```python
from build123d import *

# Parameters (mm, degrees)
SKETCH2_W           = 1006.2
SKETCH2_H           = 425
SKETCH2_W_2         = 1003.025
SKETCH2_H_2         = 421.825
BOSS_EXTRUDE1_DEPTH = 420
BOSS_EXTRUDE2_START = 420
SKETCH3_W           = 1006.2
SKETCH3_H           = 425
BOSS_EXTRUDE2_DEPTH = 1.5875
FILLET2_R           = 5
CUT_EXTRUDE1_REACH  = 1112.853
SKETCH4_W           = 80
SKETCH4_H           = 80
SKETCH7_W           = 57.15
SKETCH7_H           = 57.15
CUT_EXTRUDE2_DEPTH  = 420
SKETCH8_W           = 180
SKETCH8_H           = 100
CUT_EXTRUDE3_DEPTH  = 503.1
SKETCH9_W           = 180
SKETCH9_H           = 100
CUT_EXTRUDE4_DEPTH  = 503.1


with BuildPart() as part:
    # Sketch2 → Boss-Extrude1 (new body)
    with BuildSketch(Plane(origin=(0, 0, 0), x_dir=(1, 0, 0), z_dir=(0, 1, 0))):
        Rectangle(SKETCH2_W, SKETCH2_H)
        Rectangle(SKETCH2_W_2, SKETCH2_H_2, mode=Mode.SUBTRACT)
    extrude(amount=BOSS_EXTRUDE1_DEPTH)

    # Sketch3 → Boss-Extrude2 (add)
    with BuildSketch(Plane(origin=(0, 0, 0), x_dir=(1, 0, 0), z_dir=(0, 1, 0)).offset(BOSS_EXTRUDE2_START)):
        Rectangle(SKETCH3_W, SKETCH3_H)
    extrude(amount=-BOSS_EXTRUDE2_DEPTH)

    # Fillet2
    fillet2_edges = [part.edges().sort_by_distance(p)[0] for p in [
        (-503.1, 420, 0),
        (0, 420, 212.5),
        (503.1, 420, 0),
        (503.1, 210, 212.5),
        (-503.1, 210, 212.5),
        (-503.1, 210, -212.5),
        (503.1, 210, -212.5),
        (0, 420, -212.5),
    ]]
    fillet(fillet2_edges, radius=FILLET2_R)

    # Sketch4 → Cut-Extrude1 (cut, up to next)
    with BuildSketch(Plane.ZY.offset(503.1), mode=Mode.PRIVATE) as cut_extrude1_sk1:
        with Locations((0, 40)):
            Rectangle(SKETCH4_W, SKETCH4_H)
    cut_extrude1_tool1 = extrude(cut_extrude1_sk1.sketch, amount=-CUT_EXTRUDE1_REACH, mode=Mode.PRIVATE) & part.part
    add(cut_extrude1_tool1.solids().sort_by_distance((-503.1, 40, 0))[0], mode=Mode.SUBTRACT)

    # Sketch7 → Cut-Extrude2 (cut)
    with BuildSketch(Plane(origin=(0, 0, 0), x_dir=(1, 0, 0), z_dir=(0, 1, 0))):
        with Locations((220.4, 0)):
            Rectangle(SKETCH7_W, SKETCH7_H)
    extrude(amount=CUT_EXTRUDE2_DEPTH, mode=Mode.SUBTRACT)

    # Sketch8 → Cut-Extrude3 (cut)
    with BuildSketch(Plane(origin=(0, 0, 0), x_dir=(0, 0, -1), z_dir=(1, 0, 0))):
        with Locations((0, 330)):
            Rectangle(SKETCH8_W, SKETCH8_H)
    extrude(amount=CUT_EXTRUDE3_DEPTH, mode=Mode.SUBTRACT)

    # Sketch9 → Cut-Extrude4 (cut)
    with BuildSketch(Plane(origin=(0, 0, 0), x_dir=(0, 0, -1), z_dir=(1, 0, 0))):
        with Locations((0, 130)):
            Rectangle(SKETCH9_W, SKETCH9_H)
    extrude(amount=-CUT_EXTRUDE4_DEPTH, mode=Mode.SUBTRACT)


solid = part.part
```
Verification items for the finished model (mm, model axes). A direction names the side the tool comes from. Give positions to 0.01 mm unless a question says otherwise; leave off trailing zeros. Loops run counter-clockwise (first coordinate to the right, second up) from the corner with the lowest first, then second, coordinate; pieces in that order, holes last.
1. Section check A-A, the plane z = -74. Enter the section's corners in (x, y).
2. Section check B-B, the plane y = 139.5. Enter the section's corners in (x, z).
3. Section check D-D, the plane z = 155.5. Enter the section's corners in (x, y).
4. Thickness scan on line 1 (Z direction, x = 170.5, y = 35); line 2 (X direction, y = 65.5, z = 175); line 3 (Y direction, x = -453.5, z = -153). Record the ranges inside material, lowest first.
5. Set-up check for faces 4 (the flat face through (-7, 205, -212.5)), 5 (the flat face through (501.512, 206, 3)): record each of +Z, -Z, +X, -X, +Y, -Y from which the full face is reachable in a straight line by a thin tool's end or side.
6. Mould release check, pull along X, two halves, no side actions. Record for faces 1 (the flat face through (-7, 206, 210.912)), 2 (the flat face through (503.1, 205, 3)), 3 (the flat face through (-7, 205, 212.5)): released by +X, released by -X, zero draft, split by the parting line, or undercut.
7. Section check C-C, the plane x = -287.5. Enter the section's corners in (y, z), then the cut area to 3 significant figures.
8. Go/stop test with flat-tipped pins: pin 1 Ø0.8 at (x, z) = (502.5, -39) entering from +Y; pin 2 Ø0.8 at (x, z) = (-502, 63) entering from +Y; pin 3 Ø3 at (x, z) = (-350.5, 15) entering from -Y. Record where each tip stops, or that it passes through.
Geometry says:
1. outline: (-503.1, 0) - (-501.51, 0) - (-501.51, 80) - (-503.1, 80) - close; (-503.1, 180) - (-501.51, 180) - (-501.51, 418.41) - (501.51, 418.41) - (501.51, 380) - (503.1, 380) - (503.1, 415) arc R5 ccw to (498.1, 420) - (-498.1, 420) arc R5 ccw to (-503.1, 415) - close; (501.51, 0) - (503.1, 0) - (503.1, 280) - (501.51, 280) - close
2. outline: (-503.1, -207.5) arc R5 ccw to (-498.1, -212.5) - (498.1, -212.5) arc R5 ccw to (503.1, -207.5) - (503.1, 207.5) arc R5 ccw to (498.1, 212.5) - (-498.1, 212.5) arc R5 ccw to (-503.1, 207.5) - (-503.1, 90) - (-501.51, 90) - (-501.51, 210.91) - (501.51, 210.91) - (501.51, -210.91) - (-501.51, -210.91) - (-501.51, -90) - (-503.1, -90) - close
3. outline: (-503.1, 0) - (-501.51, 0) - (-501.51, 418.41) - (501.51, 418.41) - (501.51, 0) - (503.1, 0) - (503.1, 415) arc R5 ccw to (498.1, 420) - (-498.1, 420) arc R5 ccw to (-503.1, 415) - close
4. line 1: z = -212.5 to -210.91, 210.91 to 212.5
4. line 2: x = -503.1 to -501.51, 501.51 to 503.1
4. line 3: y = 418.41 to 420
5. face 4: -Z, +X, -X, +Y, -Y
5. face 5: -Y
6. face 1: undercut
6. face 2: released by +X
6. face 3: zero draft
7. outline: (0, -212.5) - (415, -212.5) arc R5 ccw to (420, -207.5) - (420, 207.5) arc R5 ccw to (415, 212.5) - (0, 212.5) - (0, 210.91) - (418.41, 210.91) - (418.41, -210.91) - (0, -210.91) - close
7. area: 1,990 mm2
8. pin 1: stops at y = 418
8. pin 2: stops at y = 418.57
8. pin 3: stops at y = 418.41
